```python
from build123d import *

# Parameters (mm, degrees)
SKETCH1_W           = 39
SKETCH1_H           = 39
SKETCH1_R           = 1.75
BOSS_EXTRUDE1_DEPTH = 4
SKETCH2_R           = 1.75
CUT_EXTRUDE1_DEPTH  = 11
FILLET1_R           = 1
CUT_EXTRUDE2_REACH  = 6
SKETCH3_R           = 5


with BuildPart() as part:
    # Sketch1 → Boss-Extrude1 (new body)
    with BuildSketch(Plane(origin=(0, 0, 0), x_dir=(1, 0, 0), z_dir=(0, 1, 0))):
        Rectangle(SKETCH1_W, SKETCH1_H)
        with Locations((17, 17)):
            Circle(SKETCH1_R, mode=Mode.SUBTRACT)
        with Locations((17, -17)):
            Circle(SKETCH1_R, mode=Mode.SUBTRACT)
        with Locations((-17, -17)):
            Circle(SKETCH1_R, mode=Mode.SUBTRACT)
        with Locations((-17, 17)):
            Circle(SKETCH1_R, mode=Mode.SUBTRACT)
    extrude(amount=BOSS_EXTRUDE1_DEPTH)

    # Sketch2 → Cut-Extrude1 (cut)
    with BuildSketch(Plane(origin=(0, 4, 0), x_dir=(1, 0, 0), z_dir=(0, 1, 0))):
        with Locations((10, 10)):
            Circle(SKETCH2_R)
        with Locations((10, -10)):
            Circle(SKETCH2_R)
        with Locations((-10, -10)):
            Circle(SKETCH2_R)
        with Locations((-10, 10)):
            Circle(SKETCH2_R)
    extrude(amount=-CUT_EXTRUDE1_DEPTH, mode=Mode.SUBTRACT)

    # Fillet1
    fillet1_edges = [part.edges().sort_by_distance(p)[0] for p in [
        (19.5, 2, 19.5),
        (-19.5, 2, 19.5),
        (-19.5, 2, -19.5),
        (19.5, 2, -19.5),
    ]]
    fillet(fillet1_edges, radius=FILLET1_R)

    # Sketch3 → Cut-Extrude2 (cut, up to next)
    with BuildSketch(Plane(origin=(0, 4, 0), x_dir=(1, 0, 0), z_dir=(0, 1, 0)), mode=Mode.PRIVATE) as cut_extrude2_sk1:
        Circle(SKETCH3_R)
    cut_extrude2_tool1 = extrude(cut_extrude2_sk1.sketch, amount=-CUT_EXTRUDE2_REACH, mode=Mode.PRIVATE) & part.part
    add(cut_extrude2_tool1.solids().sort_by_distance((0, 4, 0))[0], mode=Mode.SUBTRACT)


solid = part.part
```
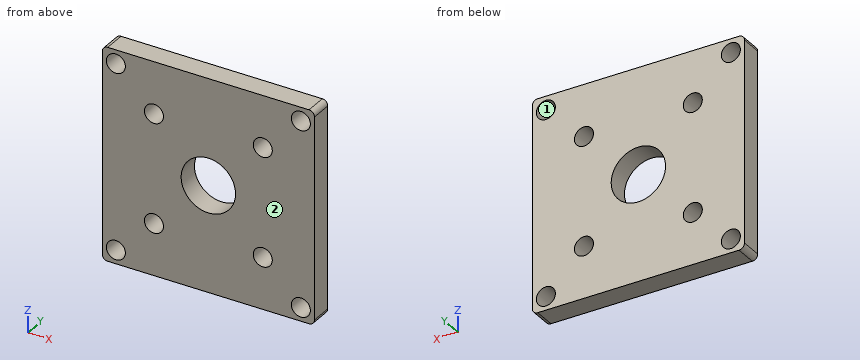
Build history of the part. All positions in model axes, mm. Face numbers are marked on the shaded views. Coordinates: 2 decimals unless noted, no trailing zeros. Order: outer loops, then holes, each group sorted by start corner. A loop starts at its lowest first (then second) coordinate and runs counter-clockwise, first axis right, second up. Notation, with made-up numbers: (10.25, 35.5) -> (44.25, 35.5) arc R36 ccw to (44.25, 69.5) -> close; hole circle Ø7 at (55, 73.25). An arc over 180 degrees is marked (long way). Answer in a Markdown table with one row per item. Add a question column.
Q1. Wall check: line 1 along Z through (x, y) = (10, 1.8); line 2 along Z through (x, y) = (-17, 1.15). Give the ranges that are in metal, low to high. Write a range as [from, to].
Q2. Band-saw the part on A-A, the plane x = 10. List the corners of the cut face in (y, z), then the cut area to 3 significant figures.
Q3. Band-saw the part on D-D, the plane y = 1.2. Give the number of separate pieces and of enclosed holes in the cut face, then the cut area to 3 significant figures.
Q4. Band-saw the part on B-B, the plane z = -10. List the corners of the cut face in (x, y), then the cut area to 3 significant figures.
Q5. Mould opens along Z. For the marked faces 1 and 2 say: +Z half, -Z half, draft (parallel to the pull), parting line (faces both ways), or undercut.
Q6. Drop a flat-ended pin along its axis: pin 1 (2 mm diameter, centred on x = -10, z = 10, fed in from -Y). Give the stop position or say it passes through.
Q7. Band-saw the part on C-C, the plane x = 0. List the corners of the cut face in (y, z), then the cut area to 3 significant figures.
Answers follow:
| question | item | result |
|---|---|---|
| 1 | line 1 | [-19.5, -11.75], [-8.25, 8.25], [11.75, 19.5] |
| 1 | line 2 | [-19.5, -18.75], [-15.25, 15.25], [18.75, 19.5] |
| 2 | outline | (0, -19.5) -> (4, -19.5) -> (4, -11.75) -> (0, -11.75) -> close; (0, -8.25) -> (4, -8.25) -> (4, 8.25) -> (0, 8.25) -> close; (0, 11.75) -> (4, 11.75) -> (4, 19.5) -> (0, 19.5) -> close |
| 2 | area | 128 mm^2 |
| 3 | separate pieces | 1 |
| 3 | enclosed holes | 9 |
| 3 | area | 1,360 mm^2 |
| 4 | outline | (-19.5, 0) -> (-11.75, 0) -> (-11.75, 4) -> (-19.5, 4) -> close; (-8.25, 0) -> (8.25, 0) -> (8.25, 4) -> (-8.25, 4) -> close; (11.75, 0) -> (19.5, 0) -> (19.5, 4) -> (11.75, 4) -> close |
| 4 | area | 128 mm^2 |
| 5 | face 1 | undercut |
| 5 | face 2 | draft |
| 6 | pin 1 | through |
| 7 | outline | (0, -19.5) -> (4, -19.5) -> (4, -5) -> (0, -5) -> close; (0, 5) -> (4, 5) -> (4, 19.5) -> (0, 19.5) -> close |
| 7 | area | 116 mm^2 |
